The model under review builds one solid part; all positions refer to its coordinate system, in mm. A direction names the side the tool comes from. Round coordinates to 2 decimals unless told otherwise and drop trailing zeros. Order: outer loops, then holes, each group sorted by start corner. A loop starts at its lowest first (then second) coordinate and runs counter-clockwise, first axis right, second up. Notation, with made-up numbers: (43.5, 43) -> (63.5, 43) arc R28 ccw to (63.5, 72) -> close; hole circle Ø11 at (18, 6.5). An arc over 180 degrees is marked (long way). Put each result on its own line as item: value. Start each with the question number.
from build123d import *

# Parameters (mm, degrees)
SKETCH1_W           = 85
SKETCH1_H           = 90
BOSS_EXTRUDE1_DEPTH = 5
SKETCH2_W           = 60
SKETCH2_H           = 26.3
CUT_EXTRUDE2_DEPTH  = 7.5
SKETCH4_W           = 5
SKETCH4_H           = 26.3
CUT_EXTRUDE3_DEPTH  = 7.5
SKETCH5_W           = 30.2
SKETCH5_H           = 5
CUT_EXTRUDE4_DEPTH  = 5
CUT_EXTRUDE5_DEPTH  = 3


with BuildPart() as part:
    # Sketch1 → Boss-Extrude1 (new body)
    with BuildSketch(Plane(origin=(0, 0, 0), x_dir=(1, 0, 0), z_dir=(0, 1, 0))):
        Rectangle(SKETCH1_W, SKETCH1_H)
    extrude(amount=BOSS_EXTRUDE1_DEPTH)

    # Sketch2 → Cut-Extrude2 (cut)
    with BuildSketch(Plane(origin=(0, 5, 0), x_dir=(1, 0, 0), z_dir=(0, 1, 0))):
        with Locations((0, -8.85)):
            Rectangle(SKETCH2_W, SKETCH2_H)
    extrude(amount=-CUT_EXTRUDE2_DEPTH, mode=Mode.SUBTRACT)

    # Sketch4 → Cut-Extrude3 (cut)
    with BuildSketch(Plane(origin=(0, 5, 0), x_dir=(1, 0, 0), z_dir=(0, 1, 0))):
        with Locations((-40, -8.85)):
            Rectangle(SKETCH4_W, SKETCH4_H)
        with Locations((40, -8.85)):
            Rectangle(SKETCH4_W, SKETCH4_H)
    extrude(amount=-CUT_EXTRUDE3_DEPTH, mode=Mode.SUBTRACT)

    # Sketch5 → Cut-Extrude4 (cut)
    with BuildSketch(Plane(origin=(0, 5, 0), x_dir=(1, 0, 0), z_dir=(0, 1, 0))):
        with Locations((0, -42.5)):
            Rectangle(SKETCH5_W, SKETCH5_H)
    extrude(amount=-CUT_EXTRUDE4_DEPTH, mode=Mode.SUBTRACT)

    # Sketch6 → Cut-Extrude5 (cut)
    with BuildSketch(Plane(origin=(0, 5, 0), x_dir=(1, 0, 0), z_dir=(0, 1, 0))):
        Polygon((-37, 35.34), (37, 35.34), (37, 24.24), (37.5, 24.24), (37.5, 18.24), (-37.5, 18.24), (-37.5, 24.24), (-37, 24.24), align=None)
    extrude(amount=-CUT_EXTRUDE5_DEPTH, mode=Mode.SUBTRACT)


solid = part.part
Q1. Take a section at B-B on y = 4.1. Give the boundary of the cut face in (x, z), and give its area (3 significant figures).
Q2. Clearance check with flat-ended pins moving along their axes: pin 1 Ø2.5 at (y, z) = (2, 13.5) entering from +X; pin 2 Ø2.5 at (y, z) = (3, 11.5) entering from -X; pin 3 Ø2.5 at (x, y) = (-2.5, 2.5) entering from +Z. State where each tip first meets the part, or that it passes through.
Q3. Take a section at D-D on z = -29. Give the boundary of the cut face in (x, y), and give its area (3 significant figures).
Q4. Take a section at A-A on x = 27.5. Give the boundary of the cut face in (y, z).
Q5. Take a section at C-C on z = 9.5. Give the boundary of the cut face in (x, y), and give its area (3 significant figures).
Q6. For faces 4 (the face through (-40, 3, 22)), 5 (the face through (0, 3, 40)), 6 (the face through (-37.5, 4, -21)), list the 3-axis set-ups (+Z, -Z, +X, -X, +Y, -Y) from which the entire face can be reached by the end or side of a thin tool; tool diameter is ignored.
Q7. Draft analysis for pull direction Z (two halves, no side actions). For faces 1 (the face through (-1, 4, -35.34)), 2 (the face through (-42.5, 2, -24)), 3 (the face through (29, 2, 45)), state which applies: +Z half, -Z half, draft (parallel to the pull), parting line (faces both ways), or undercut.
Q8. Wall thickness on probe 1 along Z at (x, y) = (28, 3.85); probe 2 along Z at (x, y) = (11, 3.15); probe 3 along X at (y, z) = (0.4, 11.5): over which ranges is each line inside the solid? List them lowest first. Write a range as [from, to].
Calculated:
1. outline: (-42.5, -45) -> (42.5, -45) -> (42.5, -4.3) -> (37.5, -4.3) -> (37.5, 22) -> (42.5, 22) -> (42.5, 45) -> (15.1, 45) -> (15.1, 40) -> (-15.1, 40) -> (-15.1, 45) -> (-42.5, 45) -> (-42.5, 22) -> (-37.5, 22) -> (-37.5, -4.3) -> (-42.5, -4.3) -> close; hole (-37.5, -24.24) -> (-37, -24.24) -> (-37, -35.34) -> (37, -35.34) -> (37, -24.24) -> (37.5, -24.24) -> (37.5, -18.24) -> (-37.5, -18.24) -> close; hole (-30, -4.3) -> (30, -4.3) -> (30, 22) -> (-30, 22) -> close
1. area: 4,390 mm²
2. pin 1: stops at x = 37.5
2. pin 2: stops at x = -37.5
2. pin 3: stops at z = 40
3. outline: (-42.5, 0) -> (42.5, 0) -> (42.5, 5) -> (37, 5) -> (37, 2) -> (-37, 2) -> (-37, 5) -> (-42.5, 5) -> close
3. area: 203 mm²
4. outline: (0, -45) -> (5, -45) -> (5, -35.34) -> (2, -35.34) -> (2, -18.24) -> (5, -18.24) -> (5, -4.3) -> (0, -4.3) -> close; (0, 22) -> (5, 22) -> (5, 45) -> (0, 45) -> close
5. outline: (-37.5, 0) -> (-30, 0) -> (-30, 5) -> (-37.5, 5) -> close; (30, 0) -> (37.5, 0) -> (37.5, 5) -> (30, 5) -> close
5. area: 75.0 mm²
6. face 4: -X, +Y, -Y
6. face 5: +Z, +Y, -Y
6. face 6: +Y
7. face 1: undercut
7. face 2: draft
7. face 3: +Z half
8. probe 1: z = [-45, -35.34], [-18.24, -4.3], [22, 45]
8. probe 2: z = [-45, -35.34], [-18.24, -4.3], [22, 40]
8. probe 3: x = [-37.5, -30], [30, 37.5]
